from build123d import *

# Parameters (mm, degrees)
F0_R     = 10
F1_DEPTH = 20
F2_R     = 10
F2_R_2   = 8
F3_DEPTH = 15.5
F5_R     = 3.75
F6_DEPTH = 25


with BuildPart() as f1:
    # F0 (on Top) → F1 (new body)
    with BuildSketch(Plane.XY):
        Circle(F0_R)
    extrude(amount=F1_DEPTH)

    # F2 (on face) → F3 (cut)
    with BuildSketch(Plane.XY.offset(20)):
        Circle(F2_R)
        Circle(F2_R_2, mode=Mode.SUBTRACT)
    extrude(amount=-F3_DEPTH, mode=Mode.SUBTRACT)

    # F5 (on offset) → F6 (cut)
    with BuildSketch(Plane.YZ.offset(10)):
        with Locations((0, 12.5)):
            Circle(F5_R)
    extrude(amount=-F6_DEPTH, mode=Mode.SUBTRACT)


solid = f1.part
Model file for the job. Use its own axes, mm. A direction names the side the tool comes from. Coordinates: 2 decimals unless noted, no trailing zeros. Write each loop counter-clockwise with the first axis right and the second up, starting at its lowest first coordinate (ties: lowest second). Pieces come first, ordered by that corner, then holes. Notation, with made-up numbers: (32.5, 36.25) -> (68.5, 36.25) arc R31 ccw to (68.5, 71.25) -> close; hole circle Ø1 at (5.25, -6.5). An arc over 180 degrees is marked (long way). One line per item, written item: value. Start each with the question number.
1) Slice it at A-A on y = 0. Write the cut outline in (x, z), then the cut area to 3 significant figures.
2) Flat gauge pins, fed straight in: pin 1 Ø4 at (x, z) = (-7, 6) entering from -Y; pin 2 Ø6 at (y, z) = (8, 15) entering from +X (3 decimals); pin 3 Ø5 at (y, z) = (5.5, 10.5) entering from -X; pin 4 Ø2 at (y, z) = (2, 13.5) entering from -X. Where does each tip first touch, or does it go through?
3) Pull direction Z, two halves, no side cores. Call faces 1 (the face through (0, 0, 0)), 2 (the face through (0, 8.2, 4.5)), 3 (the face through (0.109, -3.746, 12.665)): +Z half, -Z half, draft (parallel to the pull), parting line (faces both ways), or undercut.
4) Slice it at B-B on x = 0. Write the cut outline in (y, z).
5) Slice it at C-C on z = 15. Write the cut outline in (x, y).
6) Probe probe 1 along Z at (x, y) = (2.25, 0); probe 2 along Y at (x, z) = (0, 12.5); probe 3 along Y at (x, z) = (6.5, 14). List the from-to ranges inside material, lowest first.
7) Which spindle directions (+Z, -Z, +X, -X, +Y, -Y) get a long thin tool onto all of the face, cutting with end or side? Do faces 4 (the face through (0, 0, 20)), 5 (the face through (-6.349, -4.868, 12.358)). Say none if no direction does.
8) Slice it at D-D on z = 7. Write the cut outline in (x, y).
Answers follow:
1. outline: (-10, 0) -> (10, 0) -> (10, 4.5) -> (8, 4.5) -> (8, 8.75) -> (-8, 8.75) -> (-8, 4.5) -> (-10, 4.5) -> close; (-8, 16.25) -> (8, 16.25) -> (8, 20) -> (-8, 20) -> close
1. area: 218 mm2
2. pin 1: y = -8.23
2. pin 2: x = 6.245
2. pin 3: x = -7.41
2. pin 4: through
3. face 1: -Z half
3. face 2: +Z half
3. face 3: undercut
4. outline: (-10, 0) -> (10, 0) -> (10, 4.5) -> (8, 4.5) -> (8, 20) -> (-8, 20) -> (-8, 4.5) -> (-10, 4.5) -> close; hole circle Ø7.5 at (0, 12.5)
5. outline: (-7.5, -2.8) arc R8 ccw to (7.5, -2.8) -> close; (-7.5, 2.8) -> (7.5, 2.8) arc R8 ccw to start
6. probe 1: 0 to 8.75, 16.25 to 20
6. probe 2: -8 to -3.75, 3.75 to 8
6. probe 3: -4.66 to -3.44, 3.44 to 4.66
7. face 4: +Z, +X, -X, +Y, -Y
7. face 5: +Z
8. outline: circle Ø16 at (0, 0)
